Autodesk Inventor part; units mm, degrees
ref_plane "YZ Plane" through (0, 0, 0) normal (1, 0, 0) x (0, 1, 0)
ref_plane "XZ Plane" through (0, 0, 0) normal (0, 1, 0) x (-1, 0, 0)
ref_plane "XY Plane" through (0, 0, 0) normal (0, 0, 1) x (1, 0, 0)
sketch "Sketch1" plane through (0, 0, 0) normal (0, 1, 0) x (-1, 0, 0)
  line L0 (0, 0) -> (77, 0)
  line L1 (77, 0) -> (77, -96)
  line L2 (77, -96) -> (0, -96)
  line L3 (0, -96) -> (0, 0)
  line L4 (80, -99) -> (80, 3)
  line L5 (80, 3) -> (-3, 3)
  line L6 (-3, 3) -> (-3, -99)
  line L7 (-3, -99) -> (80, -99)
  dimension "d0" = 77
  dimension "d1" = 96
  dimension "d2" = 3
extrude "Extrusion1" add sketch "Sketch1" along normal blind 10 contours L0 L1 L2 L3 | L7 L6 L5 L4
sketch "Sketch2" plane through (0, 10, 0) normal (0, 1, 0) x (1, 0, 0)
  line L0 (0, 0) -> (-77, 0)
  line L1 (-77, 0) -> (-77, 96)
  line L2 (-77, 96) -> (0, 96)
  line L3 (0, 96) -> (0, 0)
  dimension "d5" = 77
  dimension "d6" = 96
extrude "Extrusion2" cut sketch "Sketch2" against normal blind 8
sketch "Sketch3" plane through (0, 2, 0) normal (0, 1, 0) x (1, 0, 0)
  line L0 (0, 96) -> (0, 0)
  line L1 (0, 0) -> (0, 7.5)
  line L2 (0, 7.5) -> (-7.5, 7.5)
  circle A0 centre (-7.5, 7.5) radius 1.75
  circle A1 centre (-7.5, 65.5) radius 1.75
  circle A2 centre (-56.5, 7.5) radius 1.75
  circle A3 centre (-56.5, 65.5) radius 1.75
  dimension "d9" = 7.5
  dimension "d10" = 7.5
  dimension "d11" = 3.5
  dimension "d14" = 58
  dimension "d17" = 49
extrude "Extrusion3" cut sketch "Sketch3" against normal blind 3
fillet "Fillet1" radius 5 4 edges at (-38.5, 0, 3) (-80, 0, -48) (3, 0, -48) (-38.5, 0, -99)
properties part number "MainPCB_RPI_Top"
Here's how the part is built. I have some questions about the finished solid (model axes, mm). A direction names the side the tool comes from. Round coordinates to 2 decimals unless told otherwise and drop trailing zeros. Loops run counter-clockwise (first coordinate to the right, second up) from the corner with the lowest first, then second, coordinate; pieces in that order, holes last. Notation, with made-up numbers: (89, 83) -> (129, 83) arc R32 cw to (129, 112) -> close; hole circle Ø8 at (-21, -32). An arc over 180 degrees is marked (long way). Answer as CSV lines item,"result".
1. If we section it at A-A on z = -7.5: Please give me the cut outline in (x, y).
Final values:
outline,"(-80, 5) arc R5 ccw to (-75, 0) -> (-58.25, 0) -> (-58.25, 2) -> (-77, 2) -> (-77, 10) -> (-80, 10) -> close; (-54.75, 0) -> (-9.25, 0) -> (-9.25, 2) -> (-54.75, 2) -> close; (-5.75, 0) -> (-2, 0) arc R5 ccw to (3, 5) -> (3, 10) -> (0, 10) -> (0, 2) -> (-5.75, 2) -> close"
2. Thinking about a two-plate mould opening in Z: for faces 3 (the face through (-39, 6, -96)), 4 (the face through (-5.883, 1.014, -6.83)), 5 (the face through (-38, 2, 2)), 6 (the face through (2, 10, -48)), which applies, released by +Z, released by -Z, zero draft, split by the parting line, or undercut?
Final values:
face 3,"undercut"
face 4,"undercut"
face 5,"released by +Z"
face 6,"zero draft"
3. For pin 1 (12 mm diameter, centred on x = -55, z = -67.5, fed in from +Y); pin 2 (1 mm diameter, centred on y = 2.5, z = -54, fed in from +X), each with a flat end and sliding along its axis, tell me the tip position at first contact or that it passes through.
Final values:
pin 1,"stops at y = 2"
pin 2,"stops at x = 2.58"
4. If we section it at B-B on y = 6.25: Please give me the cut outline in (x, z).
Final values:
outline,"(-80, -99) -> (3, -99) -> (3, 3) -> (-80, 3) -> close; hole (-77, -96) -> (0, -96) -> (0, 0) -> (-77, 0) -> close"
5. If we section it at D-D on z = -28: Please give me the cut outline in (x, y), plus the area to 3 significant figures.
Final values:
outline,"(-80, 5) arc R5 ccw to (-75, 0) -> (-2, 0) arc R5 ccw to (3, 5) -> (3, 10) -> (0, 10) -> (0, 2) -> (-77, 2) -> (-77, 10) -> (-80, 10) -> close"
area,"203 mm^2"
6. Which directions (+Z, -Z, +X, -X, +Y, -Y) give clear straight access to the entire face, cutting with the end or side of a thin tool? Please do faces 1 (the face through (2, 2, -49)), 2 (the face through (-39, 2, -49)).
Final values:
face 1,"+Z, -Z, +X, -Y"
face 2,"+Y"
7. If we section it at C-C on x = -7.5: Please give me the cut outline in (y, z), plus the area to 3 significant figures.
Final values:
outline,"(0, -94) arc R5 ccw to (5, -99) -> (10, -99) -> (10, -96) -> (2, -96) -> (2, -67.25) -> (0, -67.25) -> close; (0, -63.75) -> (2, -63.75) -> (2, -9.25) -> (0, -9.25) -> close; (0, -5.75) -> (2, -5.75) -> (2, 0) -> (10, 0) -> (10, 3) -> (5, 3) arc R5 ccw to (0, -2) -> close"
area,"227 mm^2"
8. If I drill on L1, parallel to Z at x = -44.5, y = 4.5; L2, parallel to X at y = 9.5, z = -57; L3, parallel to X at y = 1, z = -7.5, over which ranges is the centre line in solid material (lowest first)?
Final values:
L1,"z = -98.97 to -96, 0 to 2.97"
L2,"x = -80 to -77, 0 to 3"
L3,"x = -78 to -58.25, -54.75 to -9.25, -5.75 to 1"
